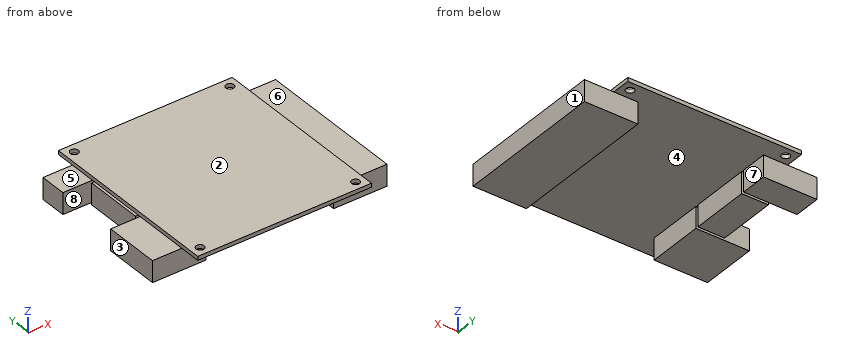
from build123d import *

# Parameters (mm, degrees)
SKETCH_1_W               = 65
SKETCH_1_H               = 70
EXTRUDE_1_DEPTH          = 1.45
SKETCH_2_R               = 1.5
CUT_EXTRUDE_1_DEPTH      = 2.45
MIRROR_2_COPY_1_SKETCH_R = 1.5
MIRROR_2_COPY_1_DEPTH    = 2.45
SKETCH_3_W               = 10
SKETCH_3_H               = 56
EXTRUDE_3_DEPTH          = 8
SKETCH_4_W               = 10
SKETCH_4_H               = 10
EXTRUDE_4_DEPTH          = 8
SKETCH_5_W               = 10
SKETCH_5_H               = 22
EXTRUDE_5_DEPTH          = 8
SKETCH_6_W               = 10
SKETCH_6_H               = 21
EXTRUDE_6_DEPTH          = 8
SKETCH_7_W               = 8
SKETCH_7_H               = 21
EXTRUDE_7_DEPTH          = 10
SKETCH_9_W               = 8
SKETCH_9_H               = 10
EXTRUDE_9_DEPTH          = 10
SKETCH_10_W              = 8
SKETCH_10_H              = 56
EXTRUDE_10_DEPTH         = 10


with BuildPart() as part:
    # 草圖1 → 填料-伸長1 (new body)
    with BuildSketch(Plane.XY):
        Rectangle(SKETCH_1_W, SKETCH_1_H)
    extrude(amount=EXTRUDE_1_DEPTH)

    # 草圖2 → 除料-伸長1 (cut, through all)
    with BuildSketch(Plane(origin=(0, 0, 0), x_dir=(-1, 0, 0), z_dir=(0, 0, -1))):
        with Locations((29.1, 31.6)):
            Circle(SKETCH_2_R)
    cut_extrude_1 = extrude(amount=-CUT_EXTRUDE_1_DEPTH, mode=Mode.SUBTRACT)

    # 鏡射1: 除料-伸長1 across plane
    add(cut_extrude_1.mirror(Plane(origin=(0, 0, 0), x_dir=(0, 0, 1), z_dir=(1, 0, 0))), mode=Mode.SUBTRACT)

    # 鏡射2: 除料-伸長1 across plane
    add(cut_extrude_1.mirror(Plane.ZX), mode=Mode.SUBTRACT)

    # 鏡射2 copy 1 sketch → 鏡射2 copy 1 (cut, through all)
    with BuildSketch(Plane(origin=(0, 0, 0), x_dir=(1, 0, 0), z_dir=(0, 0, -1))):
        with Locations((29.1, 31.6)):
            Circle(MIRROR_2_COPY_1_SKETCH_R)
    extrude(amount=-MIRROR_2_COPY_1_DEPTH, mode=Mode.SUBTRACT)

    # 草圖3 → 填料-伸長3 (add)
    with BuildSketch(Plane(origin=(0, 0, 0), x_dir=(-1, 0, 0), z_dir=(0, 0, -1))):
        with Locations((-28.5, 0)):
            Rectangle(SKETCH_3_W, SKETCH_3_H)
    extrude(amount=EXTRUDE_3_DEPTH)

    # 草圖4 → 填料-伸長4 (add)
    with BuildSketch(Plane(origin=(0, 0, 0), x_dir=(-1, 0, 0), z_dir=(0, 0, -1))):
        with Locations((28.5, 23)):
            Rectangle(SKETCH_4_W, SKETCH_4_H)
    extrude(amount=EXTRUDE_4_DEPTH)

    # 草圖5 → 填料-伸長5 (add)
    with BuildSketch(Plane(origin=(0, 0, 0), x_dir=(-1, 0, 0), z_dir=(0, 0, -1))):
        with Locations((28.5, 6)):
            Rectangle(SKETCH_5_W, SKETCH_5_H)
    extrude(amount=EXTRUDE_5_DEPTH)

    # 草圖6 → 填料-伸長6 (add)
    with BuildSketch(Plane(origin=(0, 0, 0), x_dir=(-1, 0, 0), z_dir=(0, 0, -1))):
        with Locations((28.5, -16.5)):
            Rectangle(SKETCH_6_W, SKETCH_6_H)
    extrude(amount=EXTRUDE_6_DEPTH)

    # 草圖7 → 填料-伸長7 (add)
    with BuildSketch(Plane.ZY.offset(33.5)):
        with Locations((-4, -16.5)):
            Rectangle(SKETCH_7_W, SKETCH_7_H)
    extrude(amount=EXTRUDE_7_DEPTH)

    # 草圖9 → 填料-伸長9 (add)
    with BuildSketch(Plane.ZY.offset(33.5)):
        with Locations((-4, 23)):
            Rectangle(SKETCH_9_W, SKETCH_9_H)
    extrude(amount=EXTRUDE_9_DEPTH)

    # 草圖10 → 填料-伸長10 (add)
    with BuildSketch(Plane(origin=(33.5, 0, 0), x_dir=(0, 0, -1), z_dir=(1, 0, 0))):
        with Locations((4, 0)):
            Rectangle(SKETCH_10_W, SKETCH_10_H)
    extrude(amount=EXTRUDE_10_DEPTH)


solid = part.part
Model file for the job. Use its own axes, mm. Face numbers are marked on the shaded views. A direction names the side the tool comes from. Round coordinates to 2 decimals unless told otherwise and drop trailing zeros. Order: outer loops, then holes, each group sorted by start corner. A loop starts at its lowest first (then second) coordinate and runs counter-clockwise, first axis right, second up.
(1) Pin check, flat tips, straight feed: pin 1 (3.5 mm diameter, centred on x = 29.1, y = 31.6, fed in from -Z); pin 2 (1.8 mm diameter, centred on x = 29.1, y = -31.6, fed in from +Z); pin 3 (1.5 mm diameter, centred on x = 24, z = -5, fed in from -Y); pin 4 (3.5 mm diameter, centred on x = 36, y = -6, fed in from +Z). Stop position of each tip, or through.
(2) 3-axis set-ups, long thin cutter, end or side, ignore diameter. For the marked faces 5, 6, 7 and 8: which of +Z, -Z, +X, -X, +Y, -Y reach the whole face in a straight line?
(3) Drill centre lines: line 1 (Y direction, x = 29.1, z = 0.3); line 2 (X direction, y = -31.6, z = 1.1); line 3 (X direction, y = 3, z = -3.25). Where is each one in solid material? Low to high.
(4) Band-saw the part on C-C (y = -31.6). List the corners of the cut face in (x, z), then the cut area to 4 significant figures.
(5) Band-saw the part on D-D (y = 22). List the corners of the cut face in (x, z).
(6) Band-saw the part on A-A (x = 29.1). List the corners of the cut face in (y, z), then the cut area to 3 significant figures.
(7) Band-saw the part on B-B (z = -2). List the corners of the cut face in (x, y), then the cut area to 3 significant figures.
(8) Pull direction X, two halves, no side cores. Call the marked faces 1, 2, 3 and 4: released by +X, released by -X, zero draft, split by the parting line, or undercut.
Verdict:
1. pin 1: stops at z = 0
1. pin 2: passes through
1. pin 3: stops at y = -28
1. pin 4: stops at z = 0
2. face 5: +Z, -X, +Y, -Y
2. face 6: +Z, +X, +Y, -Y
2. face 7: -Z, +Y, -Y
2. face 8: -Z, -X
3. line 1: y = -35 to -33.1, -30.1 to 30.1, 33.1 to 35
3. line 2: x = -32.5 to -30.6, -27.6 to 27.6, 30.6 to 32.5
3. line 3: x = -33.5 to -23.5, 23.5 to 43.5
4. outline: (-32.5, 0) - (-30.6, 0) - (-30.6, 1.45) - (-32.5, 1.45) - close; (-27.6, 0) - (27.6, 0) - (27.6, 1.45) - (-27.6, 1.45) - close; (30.6, 0) - (32.5, 0) - (32.5, 1.45) - (30.6, 1.45) - close
4. area: 85.55 mm2
5. outline: (-43.5, -8) - (-23.5, -8) - (-23.5, 0) - (23.5, 0) - (23.5, -8) - (43.5, -8) - (43.5, 0) - (32.5, 0) - (32.5, 1.45) - (-32.5, 1.45) - (-32.5, 0) - (-43.5, 0) - close
6. outline: (-35, 0) - (-33.1, 0) - (-33.1, 1.45) - (-35, 1.45) - close; (-30.1, 0) - (-28, 0) - (-28, -8) - (28, -8) - (28, 0) - (30.1, 0) - (30.1, 1.45) - (-30.1, 1.45) - close; (33.1, 0) - (35, 0) - (35, 1.45) - (33.1, 1.45) - close
6. area: 541 mm2
7. outline: (-43.5, -27) - (-23.5, -27) - (-23.5, -6) - (-43.5, -6) - close; (-43.5, 18) - (-23.5, 18) - (-23.5, 28) - (-43.5, 28) - close; (-33.5, -5) - (-23.5, -5) - (-23.5, 17) - (-33.5, 17) - close; (23.5, -28) - (43.5, -28) - (43.5, 28) - (23.5, 28) - close
7. area: 1,960 mm2
8. face 1: released by +X
8. face 2: zero draft
8. face 3: released by -X
8. face 4: undercut
